from build123d import *

# Parameters (mm, degrees)
SKETCH3_W               = 79.0702
SKETCH3_H               = 158.1404
SKETCH3_W_2             = 15.6718
SKETCH3_H_2             = 79.0702
CUT_EXTRUDE1_DEPTH      = 22.225
HOLE1_D                 = 13.5128
HOLE1_DEPTH             = 20.45208
HOLE1_TIP               = 3.900809359
SKETCH7_W               = 6.35
SKETCH7_H               = 12.3063
SKETCH9_R               = 4.79425
CUT_EXTRUDE2_DEPTH      = 11.75385
CUT_EXTRUDE2_DEPTH_BACK = 11.75385


with BuildPart() as part:
    # Sketch1 → Revolve1 (revolve)
    with BuildSketch(Plane.XY):
        Polygon((0, 0), (0, 18.43405), (0.762, 19.19605), (4.318, 19.19605), (5.334, 18.18005), (6.35, 18.18005), (6.35, 19.76755), (21.463, 19.76755), (22.225, 19.00555), (22.225, 0), align=None)
    revolve(axis=Axis((22.225, 0, 0), (-1, 0, 0)))

    # Sketch2 → Revolve2 (revolve)
    with BuildSketch(Plane.XY):
        Polygon((22.225, 0), (22.225, 12.7), (42.926, 12.7), (44.45, 11.176), (44.45, 0), align=None)
    revolve(axis=Axis((44.45, 0, 0), (-1, 0, 0)))

    # Sketch3 → Cut-Extrude1 (cut)
    with BuildSketch(Plane(origin=(44.45, 0, 0), x_dir=(0, 0, -1), z_dir=(1, 0, 0))):
        Rectangle(SKETCH3_W, SKETCH3_H)
        Rectangle(SKETCH3_W_2, SKETCH3_H_2, mode=Mode.SUBTRACT)
    extrude(amount=-CUT_EXTRUDE1_DEPTH, mode=Mode.SUBTRACT)

    # Hole1
    with Locations(Plane.ZY):
        with Locations((0, 0)):
            Hole(HOLE1_D / 2, depth=HOLE1_DEPTH)
            with Locations((0, 0, -(HOLE1_DEPTH + HOLE1_TIP / 2))):  # 120° drill point
                Cone(0, HOLE1_D / 2, HOLE1_TIP, mode=Mode.SUBTRACT)

    # Sketch6 → Cut-Revolve1 (revolve, cut)
    with BuildSketch(Plane(origin=(0, 0, 0), x_dir=(-1, 0, 0), z_dir=(0, 0.999847695, 0.017452406))):
        Polygon((-14.2748, 0), (-18.897793378, 0), (-18.897793378, 12.83335), (-19.114275925, 19.76755), (-14.2748, 19.76755), align=None)
    revolve(axis=Axis((14.2748, -0.344991317, 19.764539306), (0, 0.017452406, -0.999847695)), mode=Mode.SUBTRACT)

    # Sketch7 → Cut-Revolve2 (revolve, cut)
    with BuildSketch(Plane.XY):
        with Locations((3.175, 6.15315)):
            Rectangle(SKETCH7_W, SKETCH7_H)
    revolve(axis=Axis((6.35, 0, 0), (-1, 0, 0)), mode=Mode.SUBTRACT)

    # Sketch8 → Revolve3 (revolve)
    with BuildSketch(Plane.XY):
        with BuildLine():
            Line((5.267509175, 19.683381804), (6.216617928, 18.734273051))
            ThreePointArc((6.216617928, 18.734273051), (6.253815367, 18.64447049), (6.216617928, 18.554667928))
            Line((6.216617928, 18.554667928), (5.842, 18.18005))
            Line((5.842, 18.18005), (5.334, 18.18005))
            Line((5.334, 18.18005), (5.334, 17.92605))
            Line((5.334, 17.92605), (6.35, 17.92605))
            Line((6.35, 17.92605), (6.35, 18.888259175))
            Line((6.35, 18.888259175), (5.470709175, 19.76755))
            Line((5.470709175, 19.76755), (5.267509175, 19.76755))
            Line((5.267509175, 19.76755), (5.267509175, 19.683381804))
        make_face()
    revolve(axis=Axis((6.35, 0, 0), (-1, 0, 0)))

    # Sketch9 → Cut-Extrude2 (cut, two sides)
    with BuildSketch(Plane.XY) as cut_extrude2_sk:
        with Locations((34.925, 0)):
            Circle(SKETCH9_R)
    extrude(amount=CUT_EXTRUDE2_DEPTH, mode=Mode.SUBTRACT)
    extrude(cut_extrude2_sk.sketch, amount=-CUT_EXTRUDE2_DEPTH_BACK, mode=Mode.SUBTRACT)


solid = part.part
Geometry check sheet. Reference: the model listing, model coordinates, mm. A direction names the side the tool comes from. Round coordinates to 2 decimals unless told otherwise and drop trailing zeros. Loops run counter-clockwise (first coordinate to the right, second up) from the corner with the lowest first, then second, coordinate; pieces in that order, holes last. Notation, with made-up numbers: (65.5, 44) - (106.5, 44) arc R23 cw to (106.5, 59) - close; hole circle Ø8 at (77, 66). An arc over 180 degrees is marked (long way). One line per question, with ' | ' between items. Start each with the question number.
1. Cross-section at A-A on x = 23. Record the cut outline in (y, z), then the cut area to 3 significant figures.
2. Depth check by flat-ended pin: pin 1 (5 mm diameter, centred on x = 35.5, z = -8.5, fed in from -Y); pin 2 (5 mm diameter, centred on y = 4, z = -11.5, fed in from +X) (3 decimals); pin 3 (15.5 mm diameter, centred on y = 0, z = 0, fed in from -X). Enter the tip coordinate at first touch or a pass-through.
3. Draft check along Y on faces 1 (the face through (0, -4, 12)), 2 (the face through (2.6, 18.3, -5.8)), 3 (the face through (6.35, -5, 5)). Enter one of: released by +Y, released by -Y, zero draft, split by the parting line, or undercut.
4. Tool access check on faces 4 (the face through (32.7, 12.7, 0.1)), 5 (the face through (3.2, -1.6, -12.2)), 6 (the face through (32.7, -12.7, -0.1)), 7 (the face through (5.59, -3.94, 17.75)), 8 (the face through (33, -5, 7.836)). Record the directions out of +Z, -Z, +X, -X, +Y, -Y that give a thin tool (end or side, any length) a straight path to the whole face; none if there is none.
5. Scan lines: line 1 (Z direction, x = 4, y = 0); line 2 (Y direction, x = 4.5, z = 0). Record each from-to range of solid material in increasing order. Write a range as [from, to].
Taken from the geometry:
1) outline: (-9.99, -7.84) - (9.99, -7.84) arc R12.7 ccw to (9.99, 7.84) - (-9.99, 7.84) arc R12.7 ccw to start; hole circle Ø4.69 at (0, 0) | area: 354 mm²
2) pin 1: y = -11.19 | pin 2: x = 22.225 | pin 3: x = 6.35
3) face 1: zero draft | face 2: split by the parting line | face 3: undercut
4) face 4: +X, +Y | face 5: -X | face 6: +X, -Y | face 7: none | face 8: +Z, +X, +Y, -Y
5) line 1: [-19.2, -12.31], [12.31, 19.2] | line 2: [-19.01, -12.31], [12.31, 19.01]
